Autodesk Fusion 360 part; units mm, degrees
sketch "Sketch1" plane through (0, 0, 0) normal (1, 0, 0) x (0, 0, -1)
  line L0 (-21, 21) -> (21, 21)
  line L1 (21, 21) -> (21, -21)
  line L2 (21, -21) -> (-21, -21)
  line L3 (-21, -21) -> (-21, 21)
  line L4 (-11, -21) -> (7, -21)
  line L5 (7, -53) -> (-11, -53)
  line L6 (-11, -53) -> (-11, -21)
  line L7 (-21, 0) -> (21, 0) construction
  circle A0 centre (0, 0) radius 12.5
  circle A1 centre (-2, -29.5) radius 2.75
  circle A2 centre (-2, -44.5) radius 2.75
  line L8 (-2, -44.5) -> (-2, -29.5) construction
  line L9 (-16.25, 17.2) -> (-14.75, 17.2)
  arc A3 (-14.75, 13.8) -> (-14.75, 17.2) centre (-14.75, 15.5) ccw
  line L10 (-14.75, 13.8) -> (-16.25, 13.8)
  arc A4 (-16.25, 17.2) -> (-16.25, 13.8) centre (-16.25, 15.5) ccw
  line L11 (-14.75, 15.5) -> (-16.25, 15.5) construction
  line L12 (0, 20) -> (0, 2.5)
  line L13 (14.75, 13.8) -> (16.25, 13.8)
  arc A5 (16.25, 13.8) -> (16.25, 17.2) centre (16.25, 15.5) ccw
  line L14 (16.25, 17.2) -> (14.75, 17.2)
  arc A6 (14.75, 17.2) -> (14.75, 13.8) centre (14.75, 15.5) ccw
  arc A7 (-14.75, -17.2) -> (-14.75, -13.8) centre (-14.75, -15.5) ccw
  line L15 (-14.75, -13.8) -> (-16.25, -13.8)
  arc A8 (-16.25, -13.8) -> (-16.25, -17.2) centre (-16.25, -15.5) ccw
  line L16 (-16.25, -17.2) -> (-14.75, -17.2)
  arc A9 (14.75, -13.8) -> (14.75, -17.2) centre (14.75, -15.5) ccw
  line L17 (16.25, -17.2) -> (14.75, -17.2)
  arc A10 (16.25, -17.2) -> (16.25, -13.8) centre (16.25, -15.5) ccw
  line L18 (14.75, -13.8) -> (16.25, -13.8)
  line L19 (7, -53) -> (7, -21)
  point P0 (-2, -53)
  point P1 (-2, -37)
  point P2 (-15.5, 15.5)
  dimension "d1" = 42
  dimension "d4" = 42
  dimension "d8" = 25
  dimension "d9" = 5.5
  dimension "d12" = 5.5
  dimension "d13" = 15
  dimension "d28" = 1.5
  dimension "d29" = 15.5
  dimension "d30" = 15.5
  dimension "d31" = 1.7
  dimension "d32" = 32
  dimension "d33" = 18
  dimension "d34" = 16
  dimension "d35" = 2
extrude "Extrude1" add sketch "Sketch1" along normal blind 6
sketch "Sketch4" plane through (0, 0, 0) normal (-1, 0, 0) x (0, 0, 1)
  circle A0 centre (0, 0) radius 12.5
  line L0 (21, -21) -> (21, 21)
  line L1 (21, 21) -> (-21, 21)
  line L2 (-7.5, 21) -> (7.5, 21)
  line L3 (7.5, 21) -> (7.5, 39)
  line L4 (7.5, 39) -> (-7.5, 39)
  line L5 (-7.5, 39) -> (-7.5, 21)
  line L6 (-21, 21) -> (-21, -21)
  line L7 (-21, -21) -> (-7, -21)
  circle A1 centre (2, -44.5) radius 2.75
  circle A2 centre (2, -29.5) radius 2.75
  line L8 (-7, -53) -> (11, -53)
  line L9 (11, -53) -> (11, -21)
  line L10 (11, -21) -> (21, -21)
  line L11 (-7, -21) -> (-7, -53)
  arc A3 (-14.75, 13.8) -> (-14.75, 17.2) centre (-14.75, 15.5) ccw
  line L12 (-14.75, 13.8) -> (-16.25, 13.8)
  arc A4 (-16.25, 17.2) -> (-16.25, 13.8) centre (-16.25, 15.5) ccw
  line L13 (-16.25, 17.2) -> (-14.75, 17.2)
  line L14 (16.25, -17.2) -> (14.75, -17.2)
  arc A5 (14.75, -13.8) -> (14.75, -17.2) centre (14.75, -15.5) ccw
  line L15 (14.75, -13.8) -> (16.25, -13.8)
  arc A6 (16.25, -17.2) -> (16.25, -13.8) centre (16.25, -15.5) ccw
  arc A7 (-16.25, -13.8) -> (-16.25, -17.2) centre (-16.25, -15.5) ccw
  line L16 (-16.25, -13.8) -> (-14.75, -13.8)
  arc A8 (-14.75, -17.2) -> (-14.75, -13.8) centre (-14.75, -15.5) ccw
  line L17 (-14.75, -17.2) -> (-16.25, -17.2)
  arc A9 (14.75, 17.2) -> (14.75, 13.8) centre (14.75, 15.5) ccw
  line L18 (14.75, 17.2) -> (16.25, 17.2)
  arc A10 (16.25, 13.8) -> (16.25, 17.2) centre (16.25, 15.5) ccw
  line L19 (16.25, 13.8) -> (14.75, 13.8)
  point P0 (0, 21)
  dimension "d18" = 18
  dimension "d19" = 15
extrude "Extrude2" add sketch "Sketch4" against normal up to surface (6 mm away) contours L1 L2 L3 L4 L5
sketch "Sketch5" plane through (0, 0, 0) normal (-1, 0, 0) x (0, 0, 1)
  circle A0 centre (0, 0) radius 12.5
  line L0 (21, -21) -> (21, 21)
  line L1 (21, 21) -> (7.5, 21)
  line L2 (7.5, 21) -> (7.5, 39)
  line L3 (7.5, 39) -> (-7.5, 39)
  line L4 (-7.5, 39) -> (-7.5, 21)
  line L5 (-7.5, 21) -> (-21, 21)
  circle A1 centre (0, 30) radius 2.75
  line L6 (-21, 21) -> (-21, -21)
  line L7 (-21, -21) -> (-7, -21)
  circle A2 centre (2, -44.5) radius 2.75
  circle A3 centre (2, -29.5) radius 2.75
  line L8 (-7, -53) -> (11, -53)
  line L9 (11, -53) -> (11, -21)
  line L10 (11, -21) -> (21, -21)
  line L11 (-7, -21) -> (-7, -53)
  arc A4 (-14.75, 13.8) -> (-14.75, 17.2) centre (-14.75, 15.5) ccw
  line L12 (-14.75, 13.8) -> (-16.25, 13.8)
  arc A5 (-16.25, 17.2) -> (-16.25, 13.8) centre (-16.25, 15.5) ccw
  line L13 (-16.25, 17.2) -> (-14.75, 17.2)
  line L14 (16.25, -17.2) -> (14.75, -17.2)
  arc A6 (14.75, -13.8) -> (14.75, -17.2) centre (14.75, -15.5) ccw
  line L15 (14.75, -13.8) -> (16.25, -13.8)
  arc A7 (16.25, -17.2) -> (16.25, -13.8) centre (16.25, -15.5) ccw
  arc A8 (-16.25, -13.8) -> (-16.25, -17.2) centre (-16.25, -15.5) ccw
  line L16 (-16.25, -13.8) -> (-14.75, -13.8)
  arc A9 (-14.75, -17.2) -> (-14.75, -13.8) centre (-14.75, -15.5) ccw
  line L17 (-14.75, -17.2) -> (-16.25, -17.2)
  arc A10 (14.75, 17.2) -> (14.75, 13.8) centre (14.75, 15.5) ccw
  line L18 (14.75, 17.2) -> (16.25, 17.2)
  arc A11 (16.25, 13.8) -> (16.25, 17.2) centre (16.25, 15.5) ccw
  line L19 (16.25, 13.8) -> (14.75, 13.8)
  dimension "d22" = 30
  dimension "d23" = 5.5
extrude "Extrude3" cut sketch "Sketch5" against normal blind 30 contours A1
chamfer "Chamfer1" distance 3 angle 45 4 edges at (3, 21, 21) (3, -21, 21) (3, -21, -21) (3, 21, -21)
sketch "Sketch6" plane through (6, 0, 0) normal (1, 0, 0) x (0, 0, -1)
  line L0 (18, 21) -> (7.5, 21)
  line L1 (7.5, 21) -> (7.5, 39)
  line L2 (7.5, 39) -> (-7.5, 39)
  line L3 (-7.5, 39) -> (-7.5, 21)
  line L4 (-7.5, 21) -> (-18, 21)
  line L5 (-18, 21) -> (-21, 18)
  line L6 (-21, 18) -> (-21, -18)
  circle A0 centre (0, 0) radius 12.5
  circle A1 centre (0, 30) radius 2.75
  line L7 (7, -21) -> (18, -21)
  line L8 (21, -18) -> (21, 18)
  circle A2 centre (-2, -44.5) radius 2.75
  circle A3 centre (-2, -29.5) radius 2.75
  line L9 (-21, -18) -> (-18, -21)
  line L10 (-18, -21) -> (-11, -21)
  line L11 (-11, -21) -> (-11, -53)
  line L12 (-11, -53) -> (7, -53)
  line L13 (7, -53) -> (7, -21)
  line L14 (21, 18) -> (18, 21)
  line L15 (18, -21) -> (21, -18)
  arc A4 (14.75, 17.2) -> (14.75, 13.8) centre (14.75, 15.5) ccw
  line L16 (14.75, 17.2) -> (16.25, 17.2)
  arc A5 (16.25, 13.8) -> (16.25, 17.2) centre (16.25, 15.5) ccw
  line L17 (16.25, 13.8) -> (14.75, 13.8)
  line L18 (-14.75, -17.2) -> (-16.25, -17.2)
  arc A6 (-16.25, -13.8) -> (-16.25, -17.2) centre (-16.25, -15.5) ccw
  line L19 (-16.25, -13.8) -> (-14.75, -13.8)
  arc A7 (-14.75, -17.2) -> (-14.75, -13.8) centre (-14.75, -15.5) ccw
  arc A8 (16.25, -17.2) -> (16.25, -13.8) centre (16.25, -15.5) ccw
  line L20 (16.25, -17.2) -> (14.75, -17.2)
  arc A9 (14.75, -13.8) -> (14.75, -17.2) centre (14.75, -15.5) ccw
  line L21 (14.75, -13.8) -> (16.25, -13.8)
  arc A10 (-14.75, 13.8) -> (-14.75, 17.2) centre (-14.75, 15.5) ccw
  line L22 (-14.75, 13.8) -> (-16.25, 13.8)
  arc A11 (-16.25, 17.2) -> (-16.25, 13.8) centre (-16.25, 15.5) ccw
  line L23 (-16.25, 17.2) -> (-14.75, 17.2)
equation "d31 = 3.4 mm / 2"
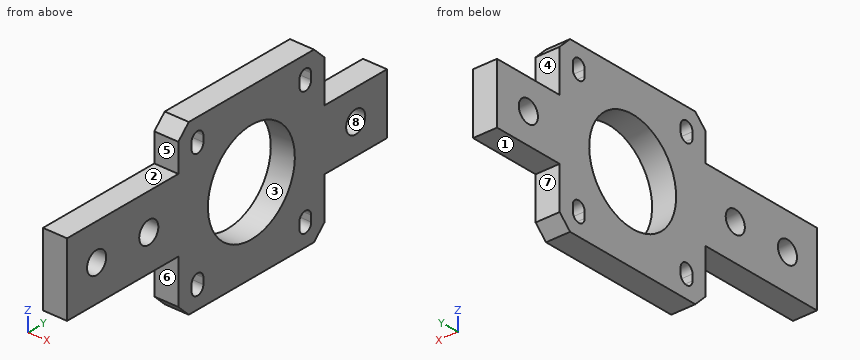
Source: CAD feature listing. Evaluate the final solid. Frame: model axes, mm. Face numbers are marked on the shaded views. A direction names the side the tool comes from. Give positions to 0.01 mm unless a question says otherwise; leave off trailing zeros. Loops run counter-clockwise (first coordinate to the right, second up) from the corner with the lowest first, then second, coordinate; pieces in that order, holes last. Notation, with made-up numbers: (38, 11.5) - (51, 11.5) arc R19 ccw to (51, 29.5) - close; hole circle Ø11 at (83, 24.25). An arc over 180 degrees is marked (long way). Use CSV: the item, a comma, the result in double quotes. Start each with the question number.
1. Pin query (flat end, axial travel): pin 1 (1.2 mm diameter, centred on x = 4.5, z = 15, fed in from -Y); pin 2 (3 mm diameter, centred on x = 2.5, y = 31, fed in from -Z); pin 3 (3 mm diameter, centred on x = 2, y = 29, fed in from +Z); pin 4 (4 mm diameter, centred on y = -41, z = -2.5, fed in from -X). Return the tip coordinate at first contact, or that it passes through.
2. Draft query along Z for the marked faces 1, 2 and 3. Return one class per face: +Z half, -Z half, draft (parallel to the pull), parting line (faces both ways), or undercut.
3. Ray query, L1, parallel to Y at x = 3.05, z = -16; L2, parallel to Y at x = 4.15, z = 0; L3, parallel to Y at x = 1.1, z = 17. Return the intervals inside material, ascending.
4. Section C-C (x = 2.25). Count the separate pieces of the cut face and the enclosed holes in it, then the cut area to 3 significant figures.
5. Section A-A (y = 0). Output: boundary loops of the cut face in (x, z).
6. Section B-B (y = 15.5). Output: boundary loops of the cut face in (x, z), then the cut area to 3 significant figures.
7. Section D-D (y = -44.5). Output: boundary loops of the cut face in (x, z).
8. Reachability of the marked faces 4, 5, 6, 7 and 8 from +Z, -Z, +X, -X, +Y, -Y: full face, straight path, thin tool, end or side. Return the list, or none.
Response:
1,pin 1,"y = -21"
1,pin 2,"z = -7.5"
1,pin 3,"z = 7.5"
1,pin 4,"x = 0"
2,face 1,"-Z half"
2,face 2,"+Z half"
2,face 3,"undercut"
3,L1,"-21 to -17.2, -13.8 to 13.8, 17.2 to 21"
3,L2,"-53 to -46.39, -42.61 to -31.39, -27.61 to -12.5, 12.5 to 27.25, 32.75 to 39"
3,L3,"-21 to -17.03, -13.97 to 13.97, 17.03 to 21"
4,separate pieces,"1"
4,enclosed holes,"8"
4,area,"1,970 mm²"
5,outline,"(0, -21) - (6, -21) - (6, -12.5) - (0, -12.5) - close; (0, 12.5) - (6, 12.5) - (6, 21) - (0, 21) - close"
6,outline,"(0, -21) - (6, -21) - (6, -17.95) - (0, -17.95) - close; (0, -13.05) - (6, -13.05) - (6, 13.05) - (0, 13.05) - close; (0, 17.95) - (6, 17.95) - (6, 21) - (0, 21) - close"
6,area,"193 mm²"
7,outline,"(0, -7) - (6, -7) - (6, -0.75) - (0, -0.75) - close; (0, 4.75) - (6, 4.75) - (6, 11) - (0, 11) - close"
8,face 4,"+Z, +X, -X, +Y"
8,face 5,"+Z, +X, -X, -Y"
8,face 6,"-Z, +X, -X, -Y"
8,face 7,"-Z, +X, -X, +Y"
8,face 8,"+X, -X"
